Answer from the drawing. Dimensions are ordinates in mm from the lowest x, y and z of the part. A direction names the side the tool comes from. Coordinates: 2 decimals unless noted, no trailing zeros. Order: outer loops, then holes, each group sorted by start corner. A loop starts at its lowest first (then second) coordinate and runs counter-clockwise, first axis right, second up. Notation, with made-up numbers: (17.25, 61) -> (40.25, 61) arc R31 cw to (40.25, 89) -> close; hole circle Ø5 at (-21, 19.25). An arc over 180 degrees is marked (long way). Answer in a Markdown table with one row per item.
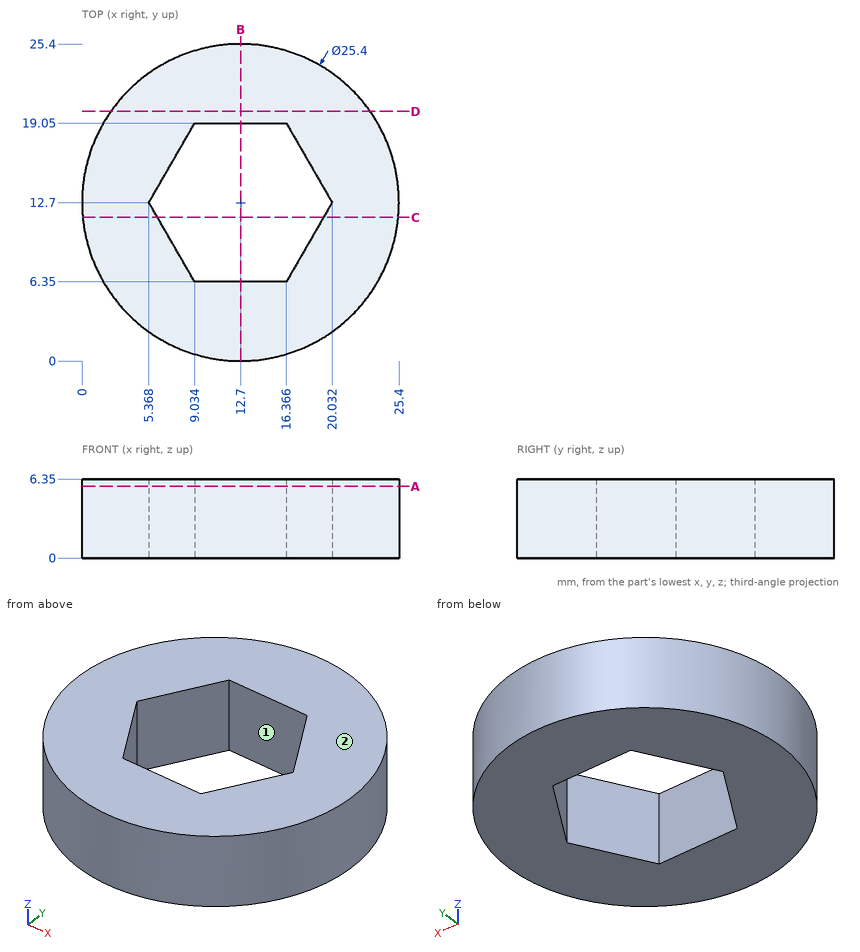
Q1. Consider line 1 (Y direction, x = 13, z = 5); line 2 (X direction, y = 10.25, z = 3.25); line 3 (X direction, y = 13, z = 5.5). Determine where each line is inside the solid, lowest interval first.
Outcome:
| item | result |
|---|---|
| line 1 | 0 to 6.35, 19.05 to 25.4 |
| line 2 | 0.24 to 6.78, 18.62 to 25.16 |
| line 3 | 0 to 5.54, 19.86 to 25.4 |
Q2. Given pin 1 (1.5 mm diameter, centred on y = 7.5, z = 2, fed in from -X) (1 decimal); pin 2 (8 mm diameter, centred on x = 15.5, y = 13, fed in from -Z); pin 3 (3 mm diameter, centred on y = 15.5, z = 5.5, fed in from -X); pin 4 (3 mm diameter, centred on x = 19.5, z = 5.5, fed in from -Y), each flat-ended and moving along its own axis, determine where each tip first touches the part or whether it passes through.
Outcome:
| item | result |
|---|---|
| pin 1 | x = 0.8 |
| pin 2 | z = 0 |
| pin 3 | x = 0.07 |
| pin 4 | y = 1.16 |
Q3. The part is cut by section A-A (z = 5.75). Write down the section's boundary in (x, y).
Outcome:
| item | result |
|---|---|
| outline | circle Ø25.4 at (12.7, 12.7); hole (5.37, 12.7) -> (9.03, 6.35) -> (16.37, 6.35) -> (20.03, 12.7) -> (16.37, 19.05) -> (9.03, 19.05) -> close |
Q4. The part is cut by section B-B (x = 12.7). Write down the section's boundary in (y, z).
Outcome:
| item | result |
|---|---|
| outline | (0, 0) -> (6.35, 0) -> (6.35, 6.35) -> (0, 6.35) -> close; (19.05, 0) -> (25.4, 0) -> (25.4, 6.35) -> (19.05, 6.35) -> close |
Q5. For the marked faces 1 and 2, determine the directions among +Z, -Z, +X, -X, +Y, -Y from which every point of the face is accessible in a straight line to the end or side of a thin tool.
Outcome:
| item | result |
|---|---|
| face 1 | +Z, -Z |
| face 2 | +Z, +X, -X, +Y, -Y |
Q6. The part is cut by section C-C (y = 11.5). Write down the section's boundary in (x, z).
Outcome:
| item | result |
|---|---|
| outline | (0.06, 0) -> (6.06, 0) -> (6.06, 6.35) -> (0.06, 6.35) -> close; (19.34, 0) -> (25.34, 0) -> (25.34, 6.35) -> (19.34, 6.35) -> close |
Q7. The part is cut by section D-D (y = 20). Write down the section's boundary in (x, z).
Outcome:
| item | result |
|---|---|
| outline | (2.31, 0) -> (23.09, 0) -> (23.09, 6.35) -> (2.31, 6.35) -> close |
